Could you check a few things on this model? Use its own coordinates, in mm. Round coordinates to 2 decimals unless told otherwise and drop trailing zeros. Order: outer loops, then holes, each group sorted by start corner. A loop starts at its lowest first (then second) coordinate and runs counter-clockwise, first axis right, second up. Notation, with made-up numbers: (14, 0) -> (42, 0) arc R6 ccw to (42, 7) -> close; hole circle Ø11 at (-2.5, -28.75). An arc over 180 degrees is marked (long way). One line per question, with ' | ' between items.
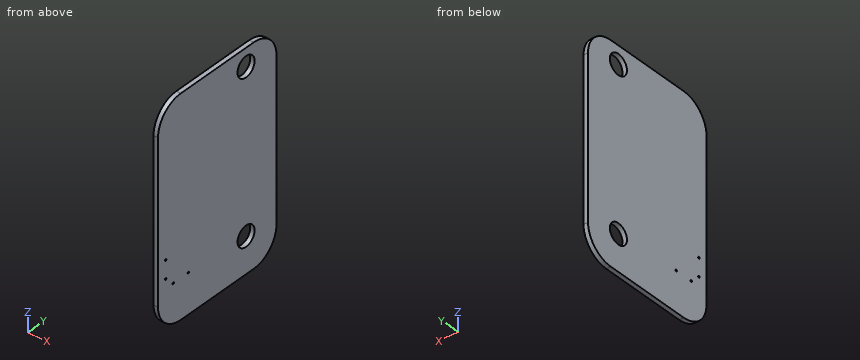
Autodesk Inventor part; units mm, degrees
ref_plane "YZ Plane" through (0, 0, 0) normal (1, 0, 0) x (0, 1, 0)
ref_plane "XZ Plane" through (0, 0, 0) normal (0, 1, 0) x (-1, 0, 0)
ref_plane "XY Plane" through (0, 0, 0) normal (0, 0, 1) x (1, 0, 0)
sketch "Sketch1" plane through (0, 0, 0) normal (1, 0, 0) x (0, 1, 0)
  line L0 (-17.3403, 309.9338) -> (-51.2615, 309.9338)
  line L1 (-51.2615, -502.8662) -> (-17.3403, -502.8662)
  line L2 (71.5597, 7.6738) -> (193.4797, 7.6738)
  line L3 (231.5797, 45.7738) -> (231.5797, 271.8338)
  line L4 (193.4797, 309.9338) -> (71.5597, 309.9338)
  line L5 (33.4597, 271.8338) -> (33.4597, 45.7738)
  line L6 (33.4597, 50.9549) -> (33.4597, 76.3549)
  line L7 (33.4597, 119.3221) -> (33.4597, 50.9549)
  arc A0 (71.5597, 309.9338) -> (33.4597, 271.8338) centre (71.5597, 271.8338) ccw
  arc A1 (231.5797, 271.8338) -> (193.4797, 309.9338) centre (193.4797, 271.8338) ccw
  arc A2 (193.4797, 7.6738) -> (231.5797, 45.7738) centre (193.4797, 45.7738) ccw
  arc A3 (33.4597, 45.7738) -> (71.5597, 7.6738) centre (71.5597, 45.7738) ccw
  circle A4 centre (180.7797, 284.5338) radius 14.2875
  circle A5 centre (46.1597, 76.3549) radius 1.27
  circle A6 centre (46.1597, 101.7549) radius 1.27
  circle A7 centre (58.8597, 63.6549) radius 1.27
  circle A8 centre (84.2597, 63.6549) radius 1.27
  circle A9 centre (180.7797, 58.4738) radius 14.2875
  point P0 (0, 0)
  dimension "d2" = 812.8
  dimension "d17" = 302.26
  dimension "d28" = 38.1
  dimension "d29" = 28.575
  dimension "d30" = 2.54
  dimension "d32" = 12.7
  dimension "d33" = 2.54
  dimension "d34" = 12.7
  dimension "d35" = 25.4
  dimension "d36" = 0
  dimension "d37" = 2.54
  dimension "d38" = 2.54
  dimension "d40" = 25.4
  dimension "d42" = 28.575
extrude "Extrusion1" add sketch "Sketch1" along normal blind 6.35
properties part number "BottomRampPlate"
1. I want a section at B-B on x = 4. List the corners of the cut face in (y, z) for me (1 decimal), and give its area (3 significant figures).
From the geometry:
outline: (33.5, 45.8) arc R38.1 ccw to (71.6, 7.7) -> (193.5, 7.7) arc R38.1 ccw to (231.6, 45.8) -> (231.6, 271.8) arc R38.1 ccw to (193.5, 309.9) -> (71.6, 309.9) arc R38.1 ccw to (33.5, 271.8) -> close; hole circle Ø2.5 at (46.2, 76.4); hole circle Ø2.5 at (46.2, 101.8); hole circle Ø2.5 at (58.9, 63.7); hole circle Ø2.5 at (84.3, 63.7); hole circle Ø28.6 at (180.8, 58.5); hole circle Ø28.6 at (180.8, 284.5) | area: 57,300 mm²
2. I want a section at A-A on y = 190. List the corners of the cut face in (x, z) for me.
From the geometry:
outline: (0, 7.67) -> (6.35, 7.67) -> (6.35, 47.56) -> (0, 47.56) -> close; (0, 69.39) -> (6.35, 69.39) -> (6.35, 273.62) -> (0, 273.62) -> close; (0, 295.45) -> (6.35, 295.45) -> (6.35, 309.93) -> (0, 309.93) -> close
3. I want a section at C-C on y = 212.5. List the corners of the cut face in (x, z) for me.
From the geometry:
outline: (0, 12.76) -> (6.35, 12.76) -> (6.35, 304.85) -> (0, 304.85) -> close
4. I'm going to push flat-ended pins straight in: pin 1 (3.5 mm diameter, centred on y = 58.86, z = 63.65, fed in from +X); pin 2 (1.5 mm diameter, centred on y = 84.26, z = 63.65, fed in from +X). Where does each tip first touch, or does it pass through?
From the geometry:
pin 1: stops at x = 6.35 | pin 2: passes through
5. I need wall thicknesses on probe 1 along Z at (x, y) = (5.75, 172); probe 2 along Z at (x, y) = (5.5, 193); probe 3 along Y at (x, z) = (5.5, 68). Which ranges of each line are inside material? Lowest first, please.
From the geometry:
probe 1: z = 7.67 to 47.2, 69.75 to 273.26, 295.81 to 309.93 | probe 2: z = 7.67 to 51.07, 65.88 to 277.13, 291.94 to 309.93 | probe 3: y = 33.46 to 170.13, 191.43 to 231.58
